from build123d import *

# Parameters (mm, degrees)
CHAMFER_SIZE = 1


with BuildPart() as part:
    # Sketch → Revolution (revolve)
    with BuildSketch(Plane.XZ):
        with BuildLine():
            Line((3, 0), (3, 17))
            Line((3, 17), (10, 17))
            Line((10, 17), (10, 28))
            Line((10, 28), (12.5, 28))
            Line((12.5, 28), (12.5, 19.5))
            ThreePointArc((12.5, 19.5), (13.232233, 17.732233), (15, 17))
            Line((15, 10), (15, 17))
            Line((7.5, 10), (15, 10))
            Line((7.5, 0), (7.5, 10))
            Line((3, 0), (7.5, 0))
        make_face()
    revolve(axis=Axis((0, 0, 0), (0, 0, 1)))

    # Chamfer
    chamfer_edges = [part.edges().sort_by_distance(p)[0] for p in [
        (-15, 0, 17),
        (-3, 0, 0),
        (-3, 0, 17),
    ]]
    chamfer(chamfer_edges, length=CHAMFER_SIZE)


solid = part.part
Source: CAD feature listing. Evaluate the final solid. Frame: model axes, mm. A direction names the side the tool comes from. Round coordinates to 2 decimals unless told otherwise and drop trailing zeros. Loops run counter-clockwise (first coordinate to the right, second up) from the corner with the lowest first, then second, coordinate; pieces in that order, holes last. Notation, with made-up numbers: (45.5, -20) -> (49.5, -20) arc R9 ccw to (49.5, -11) -> close; hole circle Ø6 at (5, 64). An arc over 180 degrees is marked (long way). Answer as a JSON object with one key per item and string values. Group by question number.
Q1. Contact query for flat-ended pins moving along their axis: P1, Ø2, axis at x = -2.5, z = 4, coming from the -Y side; P2, Ø4, axis at x = 5, y = 9.5, coming from the -Z side; P3, Ø10, axis at x = 2.5, y = 1.5, coming from the +Z side; P4, Ø3.5, axis at x = 0, y = 0, coming from the -Z side. Output: stop coordinate, or through.
Q2. Mould query, pull axis Y, two halves, no side actions, for faces 4 (the flat face through (-4.3, 0.1, 17)), 5 (the cylindrical face through (-7.493, 0.33, 5.07)), 6 (the flat face through (-3, -3, 0)). Classes: pulls with the +Y half, pulls with the -Y half, needs draft (parallel to the pull), parting line crosses it, or undercut.
Q3. Access query for faces 1 (the cylindrical face through (-3, 0, 9)), 2 (the flat face through (4, 7, 10)), 3 (the cylindrical face through (-2.17, -9.76, 22.58)). Directions: +Z, -Z, +X, -X, +Y, -Y. A direction counts if a zero-diameter tool reaches every point of the face in a straight line with its end or side. Return the directions, or none.
Q4. Section query B-B (z = 18.75). Output: boundary loops of the cut face in (x, y).
Q5. Section query A-A (z = 12.75). Output: boundary loops of the cut face in (x, y).
Q6. Ray query, line 1 (Y direction, x = 0, z = 7.5); line 2 (Y direction, x = 0, z = 24.5); line 3 (Z direction, x = 4, y = -1.5). Return the intervals inside material, ascending. Write a range as from..to.
Completed:
{
 "1": {"P1": "y = -7.35", "P2": "z = 10", "P3": "z = 17", "P4": "through"},
 "2": {"face 4": "undercut", "face 5": "parting line crosses it", "face 6": "needs draft"},
 "3": {"face 1": "+Z, -Z", "face 2": "-Z", "face 3": "+Z"},
 "4": {"outline": "circle Ø25.23 at (0, 0); hole circle Ø20 at (0, 0)"},
 "5": {"outline": "circle Ø30 at (0, 0); hole circle Ø6 at (0, 0)"},
 "6": {"line 1": "-7.5..-3, 3..7.5", "line 2": "-12.5..-10, 10..12.5", "line 3": "0..17"}
}
